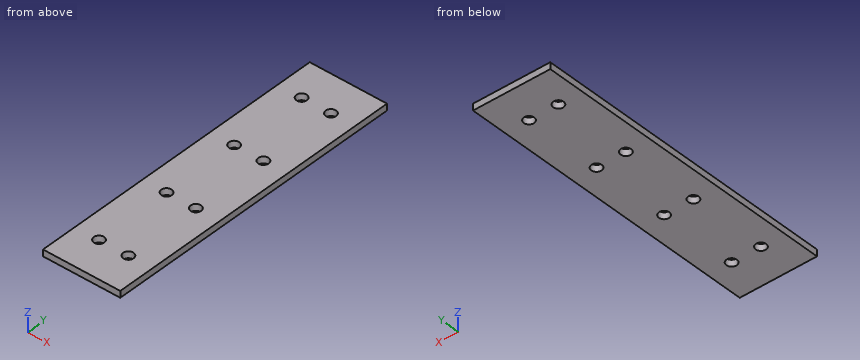
```python
from build123d import *

# Parameters (mm, degrees)
SKETCH1_W           = 20
SKETCH1_H           = 79
BOSS_EXTRUDE1_DEPTH = 1.7
SKETCH3_R           = 1.35
CUT_EXTRUDE1_DEPTH  = 41.781613504


with BuildPart() as part:
    # Sketch1 → Boss-Extrude1 (new body)
    with BuildSketch(Plane.XY):
        Rectangle(SKETCH1_W, SKETCH1_H)
    extrude(amount=BOSS_EXTRUDE1_DEPTH)

    # Sketch3 → Cut-Extrude1 (cut, through all)
    with BuildSketch(Plane.XY.offset(1.7)):
        with Locations((-3.8, 30)):
            Circle(SKETCH3_R)
        with Locations((-3.8, 10)):
            Circle(SKETCH3_R)
        with Locations((-3.8, -10)):
            Circle(SKETCH3_R)
        with Locations((-3.8, -30)):
            Circle(SKETCH3_R)
        with Locations(Location((3.8, -30, 0), (0, 0, 180))):
            Circle(SKETCH3_R)
        with Locations(Location((3.8, -10, 0), (0, 0, 180))):
            Circle(SKETCH3_R)
        with Locations(Location((3.8, 10, 0), (0, 0, 180))):
            Circle(SKETCH3_R)
        with Locations(Location((3.8, 30, 0), (0, 0, 180))):
            Circle(SKETCH3_R)
    extrude(amount=-CUT_EXTRUDE1_DEPTH, mode=Mode.SUBTRACT)


solid = part.part
```
The model under review builds one solid part; all positions refer to its coordinate system, in mm. Coordinates: 2 decimals unless noted, no trailing zeros. Write each loop counter-clockwise with the first axis right and the second up, starting at its lowest first coordinate (ties: lowest second). Pieces come first, ordered by that corner, then holes. Notation, with made-up numbers: (-20, -36) - (33, -36) arc R34 cw to (33, 2) - close; hole circle Ø1 at (61.5, -31). An arc over 180 degrees is marked (long way). Answer in a Markdown table with one row per item. Add a question column.
Q1. Consider section B-B on z = 0.5. Give the number of separate pieces and of enclosed holes in the cut face, then the cut area to 3 significant figures.
Q2. Consider section A-A on x = 3.8. Give the boundary of the cut face in (y, z).
Q3. Consider section C-C on y = 30. Give the boundary of the cut face in (x, z).
Q4. Consider section D-D on x = -3.25. Give the boundary of the cut face in (y, z), then the cut area to 3 significant figures.
Q5. Clearance check with a flat-ended pin moving along its axis: pin 1 (2.5 mm diameter, centred on x = -3.8, y = -30, fed in from +Z). State where the tip first meets the part, or that it passes through.
Q6. To check wall thickness, follow line 1 along Y through (x, z) = (-3.8, 1); line 2 along Y through (x, z) = (3.25, 1.2). State the ranges of each line that lie inside material, in increasing order. Write a range as from..to.
Answers below:
| question | item | result |
|---|---|---|
| 1 | separate pieces | 1 |
| 1 | enclosed holes | 8 |
| 1 | area | 1,530 mm² |
| 2 | outline | (-39.5, 0) - (-31.35, 0) - (-31.35, 1.7) - (-39.5, 1.7) - close; (-28.65, 0) - (-11.35, 0) - (-11.35, 1.7) - (-28.65, 1.7) - close; (-8.65, 0) - (8.65, 0) - (8.65, 1.7) - (-8.65, 1.7) - close; (11.35, 0) - (28.65, 0) - (28.65, 1.7) - (11.35, 1.7) - close; (31.35, 0) - (39.5, 0) - (39.5, 1.7) - (31.35, 1.7) - close |
| 3 | outline | (-10, 0) - (-5.15, 0) - (-5.15, 1.7) - (-10, 1.7) - close; (-2.45, 0) - (2.45, 0) - (2.45, 1.7) - (-2.45, 1.7) - close; (5.15, 0) - (10, 0) - (10, 1.7) - (5.15, 1.7) - close |
| 4 | outline | (-39.5, 0) - (-31.23, 0) - (-31.23, 1.7) - (-39.5, 1.7) - close; (-28.77, 0) - (-11.23, 0) - (-11.23, 1.7) - (-28.77, 1.7) - close; (-8.77, 0) - (8.77, 0) - (8.77, 1.7) - (-8.77, 1.7) - close; (11.23, 0) - (28.77, 0) - (28.77, 1.7) - (11.23, 1.7) - close; (31.23, 0) - (39.5, 0) - (39.5, 1.7) - (31.23, 1.7) - close |
| 4 | area | 118 mm² |
| 5 | pin 1 | through |
| 6 | line 1 | -39.5..-31.35, -28.65..-11.35, -8.65..8.65, 11.35..28.65, 31.35..39.5 |
| 6 | line 2 | -39.5..-31.23, -28.77..-11.23, -8.77..8.77, 11.23..28.77, 31.23..39.5 |
